```python
from build123d import *
from build123d.topology import SkipClean

# Parameters (mm, degrees)
SKETCH1_W               = 158
SKETCH1_H               = 90
BOSS_EXTRUDE1_DEPTH     = 26
FILLET1_R               = 6
SKETCH3_W               = 12
SKETCH3_H               = 90
CUT_EXTRUDE1_DEPTH      = 0.9
FILLET2_R               = 2
DRAFT1_ANGLE            = 6
DRAFT2_ANGLE            = 6
HOLE1_D                 = 4.6
HOLE1_DEPTH             = 26
HOLE1_TIP               = 1.381979424
CUT_EXTRUDE2_DEPTH      = 0.5
SHELL1_START            = -77.5
SHELL1_DEPTH            = 65
SHELL1_START_2          = -85.8
SHELL1_2_DEPTH          = 81.6
SHELL1_START_3          = 4.7
SHELL1_3_DEPTH          = 21.3
CUT_EXTRUDE_THIN1_DEPTH = 1


with BuildPart() as part:
    # Sketch1 → Boss-Extrude1 (new body)
    with BuildSketch(Plane(origin=(0, 0, 0), x_dir=(1, 0, 0), z_dir=(0, 1, 0))):
        with Locations((79, 45)):
            Rectangle(SKETCH1_W, SKETCH1_H)
    extrude(amount=BOSS_EXTRUDE1_DEPTH)

    # Fillet1
    fillet1_edges = [part.edges().sort_by_distance(p)[0] for p in [
        (0, 13, -90),
        (158, 13, -90),
        (158, 13, 0),
        (0, 13, 0),
    ]]
    fillet(fillet1_edges, radius=FILLET1_R)

    # Sketch3 → Cut-Extrude1 (cut)
    with BuildSketch(Plane.XZ):
        with Locations((6, -45)):
            Rectangle(SKETCH3_W, SKETCH3_H)
        with Locations((152, -45)):
            Rectangle(SKETCH3_W, SKETCH3_H)
    extrude(amount=-CUT_EXTRUDE1_DEPTH, mode=Mode.SUBTRACT)

    # Fillet2
    fillet2_edges = [part.edges().sort_by_distance(p)[0] for p in [
        (12, 0.45, -90),
        (12, 0.45, 0),
        (146, 0.45, 0),
        (146, 0.45, -90),
    ]]
    fillet(fillet2_edges, radius=FILLET2_R)

    # Draft1
    draft1_faces = [part.faces().sort_by_distance(p)[0] for p in [
        (151.922094589, 0.9, -45),
    ]]
    draft(draft1_faces, Plane(origin=(146, 0.9, 0), x_dir=(0, 0, 1), z_dir=(1, 0, 0)), DRAFT1_ANGLE)

    # Draft2
    draft2_faces = [part.faces().sort_by_distance(p)[0] for p in [
        (6.077905411, 0.9, -45),
    ]]
    draft(draft2_faces, Plane(origin=(12, 0.9, 0), x_dir=(0, 0, -1), z_dir=(-1, 0, 0)), DRAFT2_ANGLE)

    # Hole1
    with Locations(Plane(origin=(0, 0, 0), x_dir=(-1, 0, 0), z_dir=(0, -1, 0))):
        with Locations((-79, 6), (-79, 84), (-152, 6), (-152, 84), (-6, 84), (-6, 6)):
            Hole(HOLE1_D / 2, depth=HOLE1_DEPTH)
            with Locations((0, 0, -(HOLE1_DEPTH + HOLE1_TIP / 2))):  # 118° drill point
                Cone(0, HOLE1_D / 2, HOLE1_TIP, mode=Mode.SUBTRACT)

    # Sketch6 → Cut-Extrude2 (cut)
    with BuildSketch(Plane.XZ):
        with BuildLine():
            Line((72, -6), (72, -3))
            ThreePointArc((72, -3), (71.707106781, -2.292893219), (71, -2))
            Line((71, -2), (15, -2))
            ThreePointArc((15, -2), (14.292893219, -2.292893219), (14, -3))
            Line((14, -3), (14, -87))
            ThreePointArc((14, -87), (14.292893219, -87.707106781), (15, -88))
            Line((15, -88), (71, -88))
            ThreePointArc((71, -88), (71.707106781, -87.707106781), (72, -87))
            Line((72, -87), (72, -84))
            ThreePointArc((72, -84), (79, -77), (86, -84))
            Line((86, -84), (86, -87))
            ThreePointArc((86, -87), (86.292893219, -87.707106781), (87, -88))
            Line((87, -88), (143, -88))
            ThreePointArc((143, -88), (143.707106781, -87.707106781), (144, -87))
            Line((144, -87), (144, -3))
            ThreePointArc((144, -3), (143.707106781, -2.292893219), (143, -2))
            Line((143, -2), (87, -2))
            ThreePointArc((87, -2), (86.292893219, -2.292893219), (86, -3))
            Line((86, -3), (86, -6))
            ThreePointArc((86, -6), (79, -13), (72, -6))
        make_face()
    extrude(amount=-CUT_EXTRUDE2_DEPTH, mode=Mode.SUBTRACT)

    # Shell1: read off the stored shape, not the designer's step
    # Shell1 outline → Shell1 (cut)
    with BuildSketch(Plane.XY.offset(SHELL1_START)):
        Polygon((4.2, 5.942947809), (16.025858455, 4.7), (141.974141545, 4.7), (153.8, 5.942947809), (153.8, 26), (4.2, 26), align=None)
    extrude(amount=SHELL1_DEPTH, mode=Mode.SUBTRACT)

    # Shell1 2 outline → Shell1 2 (cut)
    with BuildSketch(Plane.XY.offset(SHELL1_START_2)):
        Polygon((4.2, 5.942947809), (16.025858455, 4.7), (141.974141545, 4.7), (153.8, 5.942947809), (153.8, 26), (4.2, 26), align=None)
    extrude(amount=SHELL1_2_DEPTH, mode=Mode.SUBTRACT)

    # Shell1 3 outline → Shell1 3 (add)
    with SkipClean():  # the faces are left unmerged after this step: merging them gives an invalid solid
        with BuildSketch(Plane(origin=(0, 0, 0), x_dir=(1, 0, 0), z_dir=(0, 1, 0)).offset(SHELL1_START_3)):
            with BuildLine():
                ThreePointArc((4.2, 7.431782106), (7.626345597, 7.626345597), (7.431782106, 4.2))
                Line((7.431782106, 4.2), (12.245798588, 4.2))
                ThreePointArc((12.245798588, 4.2), (10.596194078, 10.596194078), (4.2, 12.245798588))
                Line((4.2, 12.245798588), (4.2, 7.431782106))
            make_face()
            with BuildLine():
                ThreePointArc((4.568217894, 4.2), (4.373654403, 4.373654403), (4.2, 4.568217894))
                Line((4.2, 4.568217894), (4.2, 4.2))
                Line((4.2, 4.2), (4.568217894, 4.2))
            make_face()
            with BuildLine():
                Line((4.2, 82.568217894), (4.2, 77.754201412))
                ThreePointArc((4.2, 77.754201412), (10.596194078, 79.403805922), (12.245798588, 85.8))
                Line((12.245798588, 85.8), (7.431782106, 85.8))
                ThreePointArc((7.431782106, 85.8), (7.626345597, 82.373654403), (4.2, 82.568217894))
            make_face()
            with BuildLine():
                ThreePointArc((85.245798588, 4.2), (79, 12.5), (72.754201412, 4.2))
                Line((72.754201412, 4.2), (77.568217894, 4.2))
                ThreePointArc((77.568217894, 4.2), (79, 8.3), (80.431782106, 4.2))
                Line((80.431782106, 4.2), (85.245798588, 4.2))
            make_face()
            with BuildLine():
                Line((77.568217894, 85.8), (72.754201412, 85.8))
                ThreePointArc((72.754201412, 85.8), (79, 77.5), (85.245798588, 85.8))
                Line((85.245798588, 85.8), (80.431782106, 85.8))
                ThreePointArc((80.431782106, 85.8), (79, 81.7), (77.568217894, 85.8))
            make_face()
            with BuildLine():
                Line((4.2, 85.8), (4.2, 85.431782106))
                ThreePointArc((4.2, 85.431782106), (4.373654403, 85.626345597), (4.568217894, 85.8))
                Line((4.568217894, 85.8), (4.2, 85.8))
            make_face()
            with BuildLine():
                ThreePointArc((153.8, 12.245798588), (147.403805922, 10.596194078), (145.754201412, 4.2))
                Line((145.754201412, 4.2), (150.568217894, 4.2))
                ThreePointArc((150.568217894, 4.2), (150.373654403, 7.626345597), (153.8, 7.431782106))
                Line((153.8, 7.431782106), (153.8, 12.245798588))
            make_face()
            with BuildLine():
                Line((150.568217894, 85.8), (145.754201412, 85.8))
                ThreePointArc((145.754201412, 85.8), (147.403805922, 79.403805922), (153.8, 77.754201412))
                Line((153.8, 77.754201412), (153.8, 82.568217894))
                ThreePointArc((153.8, 82.568217894), (150.373654403, 82.373654403), (150.568217894, 85.8))
            make_face()
            with BuildLine():
                ThreePointArc((153.8, 4.568217894), (153.626345597, 4.373654403), (153.431782106, 4.2))
                Line((153.431782106, 4.2), (153.8, 4.2))
                Line((153.8, 4.2), (153.8, 4.568217894))
            make_face()
            with BuildLine():
                Line((153.8, 85.8), (153.431782106, 85.8))
                ThreePointArc((153.431782106, 85.8), (153.626345597, 85.626345597), (153.8, 85.431782106))
                Line((153.8, 85.431782106), (153.8, 85.8))
            make_face()
        extrude(amount=SHELL1_3_DEPTH)

    # Sketch7 → Cut-Extrude-Thin1 (cut)
    with SkipClean():  # the faces are left unmerged after this step: merging them gives an invalid solid
        with BuildSketch(Plane(origin=(0, 26, 0), x_dir=(1, 0, 0), z_dir=(0, 1, 0))):
            with BuildLine():
                ThreePointArc((10.530161934, 85.04887218), (9.288046533, 80.711953467), (4.95112782, 79.469838066))
                ThreePointArc((4.95112782, 79.469838066), (3.255463066, 79.086989132), (2.5, 77.52138132))
                Line((2.5, 77.52138132), (2.5, 12.47861868))
                ThreePointArc((2.5, 12.47861868), (3.255463066, 10.913010868), (4.95112782, 10.530161934))
                ThreePointArc((4.95112782, 10.530161934), (9.288046533, 9.288046533), (10.530161934, 4.95112782))
                ThreePointArc((10.530161934, 4.95112782), (10.913010868, 3.255463066), (12.47861868, 2.5))
                Line((12.47861868, 2.5), (72.52138132, 2.5))
                ThreePointArc((72.52138132, 2.5), (74.086989132, 3.255463066), (74.469838066, 4.95112782))
                ThreePointArc((74.469838066, 4.95112782), (79, 10.65), (83.530161934, 4.95112782))
                ThreePointArc((83.530161934, 4.95112782), (83.913010868, 3.255463066), (85.47861868, 2.5))
                Line((85.47861868, 2.5), (145.52138132, 2.5))
                ThreePointArc((145.52138132, 2.5), (147.086989132, 3.255463066), (147.469838066, 4.95112782))
                ThreePointArc((147.469838066, 4.95112782), (148.711953467, 9.288046533), (153.04887218, 10.530161934))
                ThreePointArc((153.04887218, 10.530161934), (154.744536934, 10.913010868), (155.5, 12.47861868))
                Line((155.5, 12.47861868), (155.5, 77.52138132))
                ThreePointArc((155.5, 77.52138132), (154.744536934, 79.086989132), (153.04887218, 79.469838066))
                ThreePointArc((153.04887218, 79.469838066), (148.711953467, 80.711953467), (147.469838066, 85.04887218))
                ThreePointArc((147.469838066, 85.04887218), (147.086989132, 86.744536934), (145.52138132, 87.5))
                Line((145.52138132, 87.5), (85.47861868, 87.5))
                ThreePointArc((85.47861868, 87.5), (83.913010868, 86.744536934), (83.530161934, 85.04887218))
                ThreePointArc((83.530161934, 85.04887218), (79, 79.35), (74.469838066, 85.04887218))
                ThreePointArc((74.469838066, 85.04887218), (74.086989132, 86.744536934), (72.52138132, 87.5))
                Line((72.52138132, 87.5), (12.47861868, 87.5))
                ThreePointArc((12.47861868, 87.5), (10.913010868, 86.744536934), (10.530161934, 85.04887218))
            make_face()
            with BuildLine():
                ThreePointArc((11.504390307, 85.27443609), (9.995153314, 80.004846686), (4.72556391, 78.495609693))
                ThreePointArc((4.72556391, 78.495609693), (3.877731533, 78.304185226), (3.5, 77.52138132))
                Line((3.5, 77.52138132), (3.5, 12.47861868))
                ThreePointArc((3.5, 12.47861868), (3.877731533, 11.695814774), (4.72556391, 11.504390307))
                ThreePointArc((4.72556391, 11.504390307), (9.995153314, 9.995153314), (11.504390307, 4.72556391))
                ThreePointArc((11.504390307, 4.72556391), (11.695814774, 3.877731533), (12.47861868, 3.5))
                Line((12.47861868, 3.5), (72.52138132, 3.5))
                ThreePointArc((72.52138132, 3.5), (73.304185226, 3.877731533), (73.495609693, 4.72556391))
                ThreePointArc((73.495609693, 4.72556391), (79, 11.65), (84.504390307, 4.72556391))
                ThreePointArc((84.504390307, 4.72556391), (84.695814774, 3.877731533), (85.47861868, 3.5))
                Line((85.47861868, 3.5), (145.52138132, 3.5))
                ThreePointArc((145.52138132, 3.5), (146.304185226, 3.877731533), (146.495609693, 4.72556391))
                ThreePointArc((146.495609693, 4.72556391), (148.004846686, 9.995153314), (153.27443609, 11.504390307))
                ThreePointArc((153.27443609, 11.504390307), (154.122268467, 11.695814774), (154.5, 12.47861868))
                Line((154.5, 12.47861868), (154.5, 77.52138132))
                ThreePointArc((154.5, 77.52138132), (154.122268467, 78.304185226), (153.27443609, 78.495609693))
                ThreePointArc((153.27443609, 78.495609693), (148.004846686, 80.004846686), (146.495609693, 85.27443609))
                ThreePointArc((146.495609693, 85.27443609), (146.304185226, 86.122268467), (145.52138132, 86.5))
                Line((145.52138132, 86.5), (85.47861868, 86.5))
                ThreePointArc((85.47861868, 86.5), (84.695814774, 86.122268467), (84.504390307, 85.27443609))
                ThreePointArc((84.504390307, 85.27443609), (79, 78.35), (73.495609693, 85.27443609))
                ThreePointArc((73.495609693, 85.27443609), (73.304185226, 86.122268467), (72.52138132, 86.5))
                Line((72.52138132, 86.5), (12.47861868, 86.5))
                ThreePointArc((12.47861868, 86.5), (11.695814774, 86.122268467), (11.504390307, 85.27443609))
            make_face(mode=Mode.SUBTRACT)
        extrude(amount=-CUT_EXTRUDE_THIN1_DEPTH, mode=Mode.SUBTRACT)


solid = part.part
```
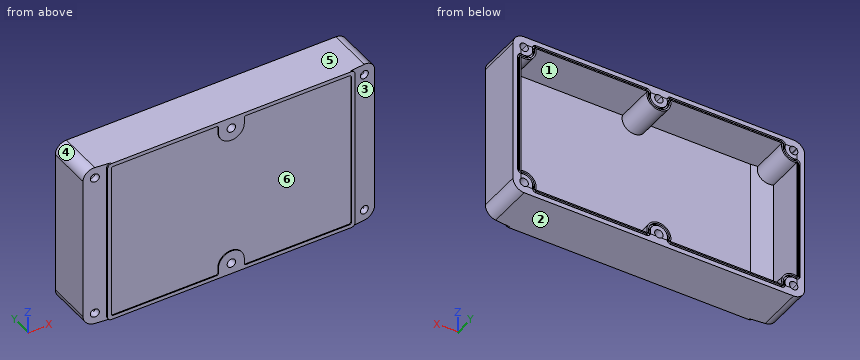
Check sheet for the modelled part. Datum: model origin and axes. Units: mm. Face numbers are marked on the shaded views. A direction names the side the tool comes from. Round coordinates to 2 decimals unless told otherwise and drop trailing zeros. Loops run counter-clockwise (first coordinate to the right, second up) from the corner with the lowest first, then second, coordinate; pieces in that order, holes last. Notation, with made-up numbers: (61.25, 52.25) -> (68.25, 52.25) arc R25 cw to (68.25, 84.25) -> close; hole circle Ø8 at (48, 30). An arc over 180 degrees is marked (long way). Answer in a Markdown table with one row per item.
Q1. Go/stop test with flat-tipped pins: P1, Ø1, axis at x = 79, z = -56, coming from the -Y side; P2, Ø0.6, axis at y = 0.5, z = -5, coming from the -X side. Record where each tip stops, or that it passes through.
Data:
| item | result |
|---|---|
| P1 | stops at y = 0.5 |
| P2 | stops at x = 12 |
Q2. Thickness scan on L1, parallel to Z at x = 152, y = 5.1; L2, parallel to X at y = 12.75, z = -84; L3, parallel to Z at x = 152, y = 10.75. Record the ranges inside material, lowest first.
Data:
| item | result |
|---|---|
| L1 | z = -90 to -86.3, -81.7 to -8.3, -3.7 to 0 |
| L2 | x = 0 to 3.7, 8.3 to 12.5, 72.5 to 76.7, 81.3 to 85.5, 145.5 to 149.7, 154.3 to 158 |
| L3 | z = -90 to -86.3, -81.7 to -77.5, -12.5 to -8.3, -3.7 to 0 |
Q3. Sectioned sample at A-A on z = -37. Enter the section's corners in (x, y), then the cut area to 3 significant figures.
Data:
| item | result |
|---|---|
| outline | (0, 2.16) -> (12, 0.9) -> (12, 0) -> (14, 0) -> (14, 0.5) -> (144, 0.5) -> (144, 0) -> (146, 0) -> (146, 0.9) -> (158, 2.16) -> (158, 26) -> (155.5, 26) -> (155.5, 25) -> (154.5, 25) -> (154.5, 26) -> (153.8, 26) -> (153.8, 5.94) -> (141.97, 4.7) -> (16.03, 4.7) -> (4.2, 5.94) -> (4.2, 26) -> (3.5, 26) -> (3.5, 25) -> (2.5, 25) -> (2.5, 26) -> (0, 26) -> close |
| area | 832 mm^2 |
Q4. Set-up check for the marked faces 1 and 2: record each of +Z, -Z, +X, -X, +Y, -Y from which the full face is reachable in a straight line by a thin tool's end or side.
Data:
| item | result |
|---|---|
| face 1 | +Y |
| face 2 | -Z, +X, -X, +Y, -Y |
Q5. Sectioned sample at B-B on x = 57. Enter the section's corners in (y, z).
Data:
| item | result |
|---|---|
| outline | (0, -90) -> (26, -90) -> (26, -87.5) -> (25, -87.5) -> (25, -86.5) -> (26, -86.5) -> (26, -85.8) -> (4.7, -85.8) -> (4.7, -4.2) -> (26, -4.2) -> (26, -3.5) -> (25, -3.5) -> (25, -2.5) -> (26, -2.5) -> (26, 0) -> (0, 0) -> (0, -2) -> (0.5, -2) -> (0.5, -88) -> (0, -88) -> close |
Q6. Release check for a two-part mould opening along X. For the marked faces 3, 4, 5 and 6 record: released by +X, released by -X, zero draft, split by the parting line, or undercut.
Data:
| item | result |
|---|---|
| face 3 | released by +X |
| face 4 | released by -X |
| face 5 | zero draft |
| face 6 | undercut |
